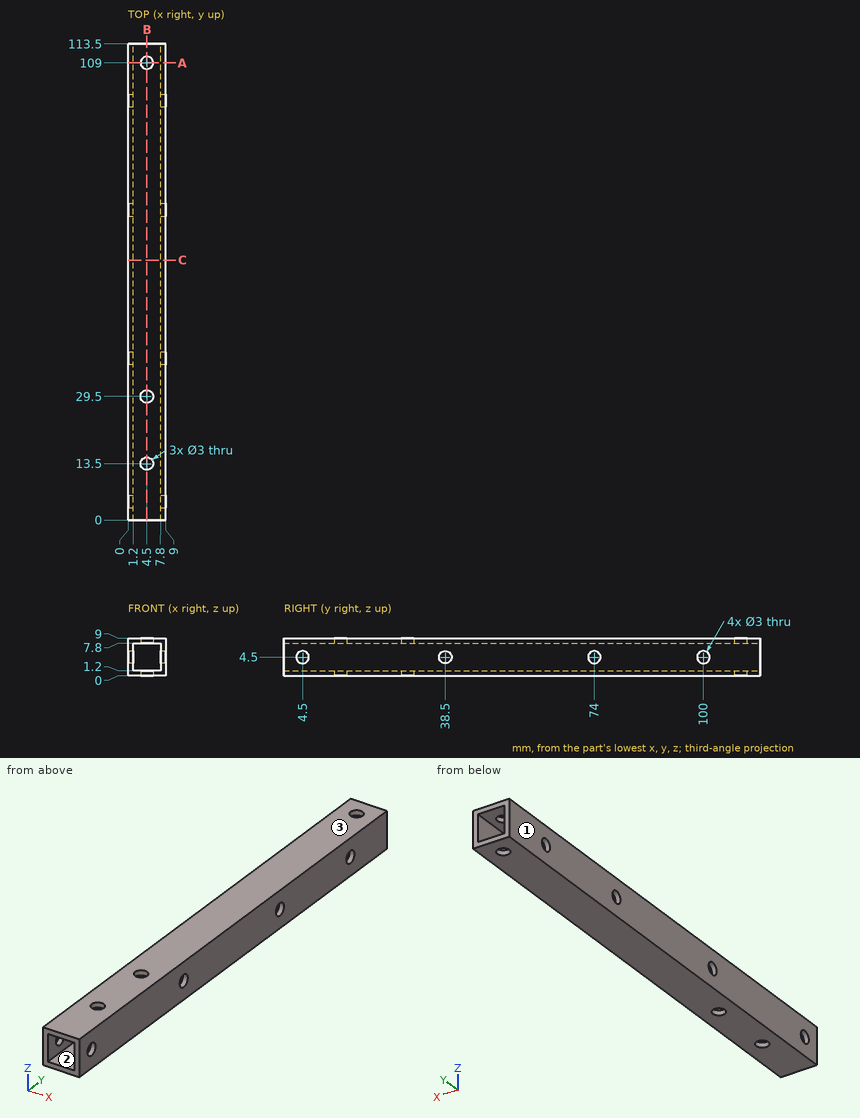
Print and shaded views of the part. All mm, measured from the part's lowest x, y and z. Coordinates: 2 decimals unless noted, no trailing zeros. Order: outer loops, then holes, each group sorted by start corner. A loop starts at its lowest first (then second) coordinate and runs counter-clockwise, first axis right, second up.
Item 1: Saw through at B-B on x = 4.5. State how many separate pieces and enclosed holes the cut face has, then the cut area to 3 significant figures.
Filled in:
separate pieces: 8
enclosed holes: 0
area: 251 mm2
Item 2: Saw through at C-C on y = 62. List the corners of the cut face in (x, z), then the cut area to 3 significant figures.
Filled in:
outline: (0, 0) - (9, 0) - (9, 9) - (0, 9) - close; hole (1.2, 1.2) - (7.8, 1.2) - (7.8, 7.8) - (1.2, 7.8) - close
area: 37.4 mm2
Item 3: Mould opens along Z. For the marked faces 1, 2 and 3 say: released by +Z, released by -Z, zero draft, split by the parting line, or undercut.
Filled in:
face 1: zero draft
face 2: undercut
face 3: released by +Z
Item 4: Drill centre lines: L1, parallel to Y at x = 0.8, z = 4.5; L2, parallel to Y at x = 4.5, z = 8.3; L3, parallel to X at y = 93, z = 5.25. Where is each one in solid material? Low to high.
Filled in:
L1: y = 0 to 3, 6 to 37, 40 to 72.5, 75.5 to 98.5, 101.5 to 113.5
L2: y = 0 to 12, 15 to 28, 31 to 107.5, 110.5 to 113.5
L3: x = 0 to 1.2, 7.8 to 9
Item 5: Saw through at A-A on y = 109. List the corners of the cut face in (x, z), then the cut area to 3 significant figures.
Filled in:
outline: (0, 0) - (3, 0) - (3, 1.2) - (1.2, 1.2) - (1.2, 7.8) - (3, 7.8) - (3, 9) - (0, 9) - close; (6, 0) - (9, 0) - (9, 9) - (6, 9) - (6, 7.8) - (7.8, 7.8) - (7.8, 1.2) - (6, 1.2) - close
area: 30.2 mm2
